Could you check a few things on this model? Use its own coordinates, in mm. Face numbers are marked on the shaded views. A direction names the side the tool comes from. Coordinates: 2 decimals unless noted, no trailing zeros. Loops run counter-clockwise (first coordinate to the right, second up) from the corner with the lowest first, then second, coordinate; pieces in that order, holes last.
from build123d import *

# Parameters (mm, degrees)
SKETCH2_W           = 10
SKETCH2_H           = 5
BOSS_EXTRUDE2_DEPTH = 10
SKETCH3_R           = 1.4
BOSS_EXTRUDE3_DEPTH = 1.8
SKETCH4_W           = 1.85
SKETCH4_H           = 0.35
CUT_EXTRUDE1_DEPTH  = 5
SKETCH5_R           = 1.2
CUT_EXTRUDE2_DEPTH  = 3.5
FILLET1_R           = 0.7


with BuildPart() as part:
    # Sketch2 → Boss-Extrude2 (new body)
    with BuildSketch(Plane(origin=(0, 0, 0), x_dir=(1, 0, 0), z_dir=(0, 1, 0))):
        with Locations((5, 2.5)):
            Rectangle(SKETCH2_W, SKETCH2_H)
    extrude(amount=BOSS_EXTRUDE2_DEPTH)

    # Sketch3 → Boss-Extrude3 (add)
    with BuildSketch(Plane(origin=(0, 0, -5), x_dir=(-1, 0, 0), z_dir=(0, 0, -1))):
        with Locations(Location((-8, 8, 0), (0, 0, 180))):
            Circle(SKETCH3_R)
        with Locations(Location((-2, 8, 0), (0, 0, 180))):
            Circle(SKETCH3_R)
    extrude(amount=BOSS_EXTRUDE3_DEPTH)

    # Sketch4 → Cut-Extrude1 (cut)
    with BuildSketch(Plane.XZ):
        with Locations((3.425, -4.825)):
            Rectangle(SKETCH4_W, SKETCH4_H)
        with Locations((6.575, -4.825)):
            Rectangle(SKETCH4_W, SKETCH4_H)
    extrude(amount=-CUT_EXTRUDE1_DEPTH, mode=Mode.SUBTRACT)

    # Sketch5 → Cut-Extrude2 (cut)
    with BuildSketch(Plane.XZ):
        with Locations(Location((5, -2.5, 0), (0, 0, 270))):
            Circle(SKETCH5_R)
    extrude(amount=-CUT_EXTRUDE2_DEPTH, mode=Mode.SUBTRACT)

    # Fillet1
    fillet1_edges = [part.edges().sort_by_distance(p)[0] for p in [
        (10, 10, -2.5),
        (0, 10, -2.5),
        (10, 0, -2.5),
        (0, 0, -2.5),
    ]]
    fillet(fillet1_edges, radius=FILLET1_R)


solid = part.part
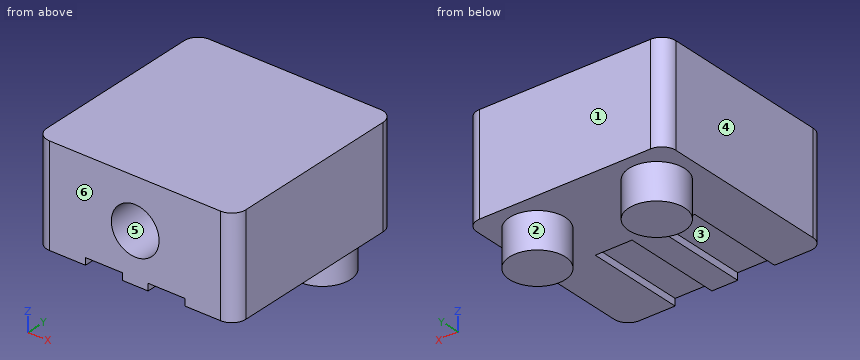
1) Will these pins go through, and if not, where does the flat tip stop? pin 1 (3 mm diameter, centred on x = 1.5, y = 3, fed in from -Z); pin 2 (0.6 mm diameter, centred on x = 3.5, y = 3, fed in from -Z).
2) Imagine slicing it at C-C on z = -2.5. List the corners of the cut face in (x, y) for me.
3) Imagine slicing it at B-B on x = 2. List the corners of the cut face in (y, z) for me, plus the area to 3 significant figures.
4) Imagine slicing it at A-A on y = 2. List the corners of the cut face in (x, z) for me.
5) Imagine slicing it at D-D on y = 8. List the corners of the cut face in (x, z) for me, plus the area to 3 significant figures.
6) We'd pull the mould along X, two halves only. Please class the marked faces 4, 5 and 6: released by +X, released by -X, zero draft, split by the parting line, or undercut.
7) If I drill on L1, parallel to X at y = 1.1, z = -2.5; L2, parallel to Z at x = 3.75, y = 6; L3, parallel to Z at x = 2.75, y = 2.25, over which ranges is the centre line in solid material (lowest first)?
8) For the marked faces 1, 2 and 3, which set-ups out of +Z, -Z, +X, -X, +Y, -Y let a thin tool reach every point of the face, with its end or its side?
Solved:
1. pin 1: stops at z = -5
1. pin 2: stops at z = -4.65
2. outline: (0, 0.7) arc R0.7 ccw to (0.7, 0) - (3.8, 0) - (3.8, 3.5) - (6.2, 3.5) - (6.2, 0) - (9.3, 0) arc R0.7 ccw to (10, 0.7) - (10, 9.3) arc R0.7 ccw to (9.3, 10) - (0.7, 10) arc R0.7 ccw to (0, 9.3) - close
3. outline: (0, -5) - (6.6, -5) - (6.6, -6.8) - (9.4, -6.8) - (9.4, -5) - (10, -5) - (10, 0) - (0, 0) - close
3. area: 55.0 mm2
4. outline: (0, -5) - (2.5, -5) - (2.5, -4.65) - (4.35, -4.65) - (4.35, -5) - (5.65, -5) - (5.65, -4.65) - (7.5, -4.65) - (7.5, -5) - (10, -5) - (10, 0) - (0, 0) - close; hole circle Ø2.4 at (5, -2.5)
5. outline: (0, -5) - (0.6, -5) - (0.6, -6.8) - (3.4, -6.8) - (3.4, -5) - (6.6, -5) - (6.6, -6.8) - (9.4, -6.8) - (9.4, -5) - (10, -5) - (10, 0) - (0, 0) - close
5. area: 60.1 mm2
6. face 4: released by -X
6. face 5: undercut
6. face 6: zero draft
7. L1: x = 0 to 3.8, 6.2 to 10
7. L2: z = -5 to 0
7. L3: z = -4.65 to 0
8. face 1: +Z, -Z, +X, -X, +Y
8. face 2: -Z
8. face 3: -Z, -Y
